Geometry: see drawing. Coordinates: mm, zero at the bounding-box minimum. A direction names the side the tool comes from. Round coordinates to 2 decimals unless told otherwise and drop trailing zeros. Write each loop counter-clockwise with the first axis right and the second up, starting at its lowest first coordinate (ties: lowest second). Pieces come first, ordered by that corner, then holes.
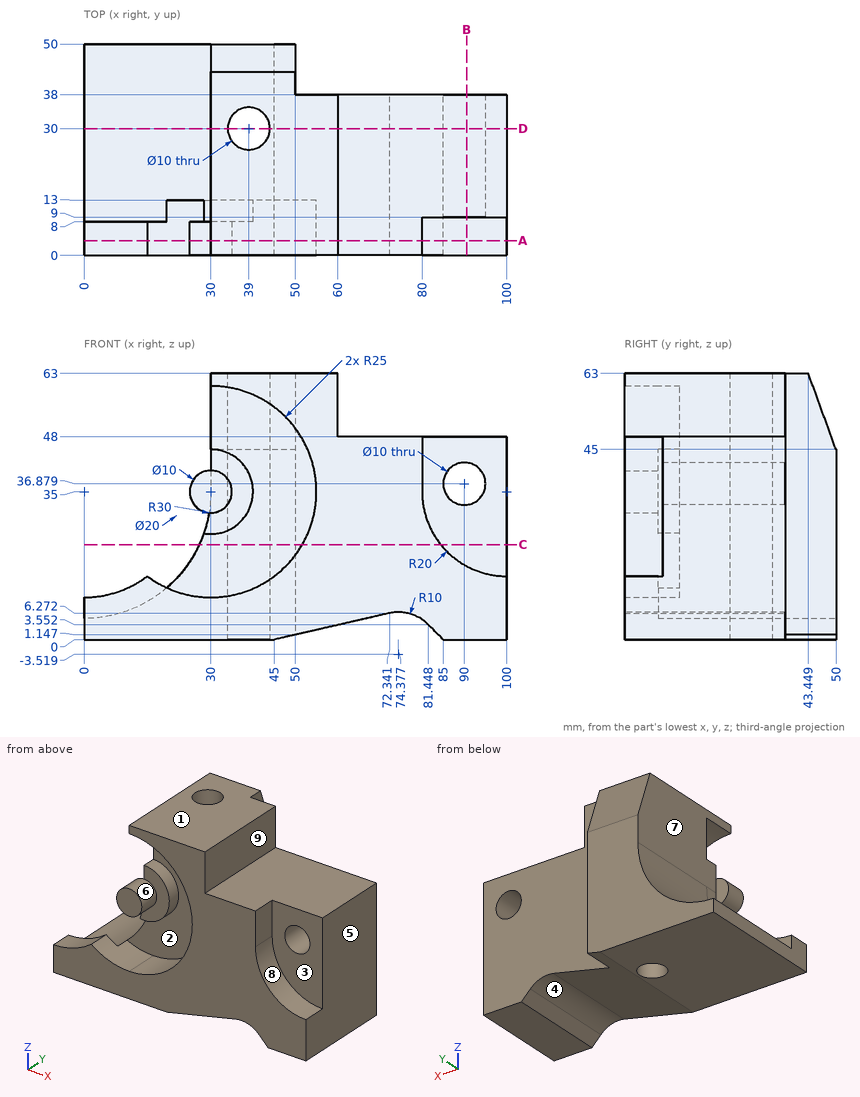
1) Pull-direction query (Z, two-part tool) for the marked faces 1, 2, 3 and 4; classes: released by +Z, released by -Z, zero draft, split by the parting line, or undercut.
Taken from the geometry:
face 1: released by +Z
face 2: undercut
face 3: zero draft
face 4: released by -Z
2) Section query A-A on y = 3.5. Return the cut outline in (x, z).
Taken from the geometry:
outline: (0, 0) - (45, 0) - (72.34, 6.27) arc R10 cw to (81.45, 3.55) - (85, 0) - (100, 0) - (100, 15) arc R20 cw to (80, 35) - (80, 48) - (60, 48) - (60, 63) - (30, 63) - (30, 60) arc R25 cw (long way) to (15, 15) arc R25 cw to (0, 10) - close; circle Ø10 at (30, 35)
3) Reachability of the marked faces 5, 6, 7, 8 and 9 from +Z, -Z, +X, -X, +Y, -Y: full face, straight path, thin tool, end or side. Return the list, or none.
Taken from the geometry:
face 5: +Z, -Z, +X, +Y, -Y
face 6: -Y
face 7: +Z, -X, +Y
face 8: +Z, +X, -Y
face 9: +Z, +X, +Y, -Y
4) Section query D-D on y = 30. Return the cut outline in (x, z), then the cut area to 3 significant figures.
Taken from the geometry:
outline: (0, 0) - (34, 0) - (34, 63) - (30, 63) - (30, 35) arc R30 cw to (0, 5) - close; (44, 0) - (45, 0) - (72.34, 6.27) arc R10 cw to (81.45, 3.55) - (85, 0) - (100, 0) - (100, 48) - (60, 48) - (60, 63) - (44, 63) - close; hole circle Ø10 at (90, 36.88)
area: 3,300 mm2
5) Material intervals for line 1 (Z direction, x = 90, y = 28); line 2 (X direction, y = 43, z = 41.5); line 3 (Y direction, x = 78.5, z = 32.5), sorted ascending.
Taken from the geometry:
line 1: z = 0 to 31.88, 41.88 to 48
line 2: x = 30 to 50
line 3: y = 0 to 38
6) Section query B-B on x = 90.5. Return the cut outline in (y, z) (1 decimal), then the cut area to 3 significant figures.
Taken from the geometry:
outline: (0, 0) - (38, 0) - (38, 31.9) - (9, 31.9) - (9, 17.4) - (0, 17.4) - close; (9, 41.9) - (38, 41.9) - (38, 48) - (9, 48) - close
area: 1,260 mm2
7) Contact query for flat-ended pins moving along their axis: P1, Ø12, axis at y = 20, z = 55, coming from the +X side; P2, Ø13, axis at x = 90, z = 36.88, coming from the +Y side; P3, Ø4, axis at y = 5.5, z = 21, coming from the +X side. Output: stop coordinate, or through.
Taken from the geometry:
P1: stops at x = 60
P2: stops at y = 38
P3: stops at x = 88
8) Section query C-C on z = 22.5. Return the cut outline in (x, y), then the cut area to 3 significant figures.
Taken from the geometry:
outline: (27.27, 13) - (51.65, 13) - (51.65, 0) - (84.39, 0) - (84.39, 9) - (100, 9) - (100, 38) - (50, 38) - (50, 50) - (27.27, 50) - close; hole circle Ø10 at (39, 30)
area: 2,500 mm2
